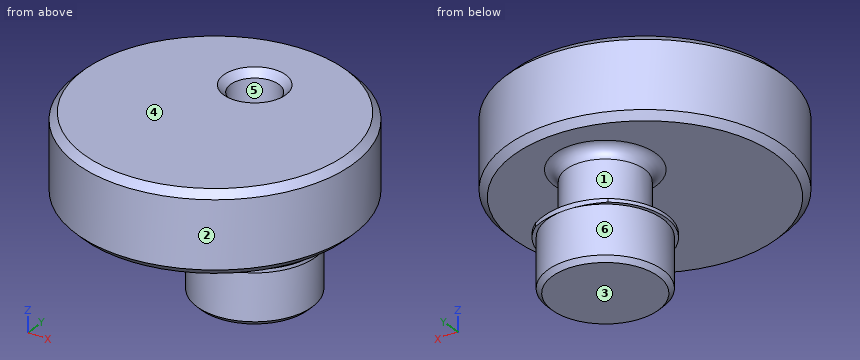
Autodesk Inventor part; units mm, degrees
ref_plane "YZ Plane" through (0, 0, 0) normal (1, 0, 0) x (0, 1, 0)
ref_plane "XZ Plane" through (0, 0, 0) normal (0, 1, 0) x (-1, 0, 0)
ref_plane "XY Plane" through (0, 0, 0) normal (0, 0, 1) x (1, 0, 0)
sketch "Sketch1" plane through (0, 0, 0) normal (0, 0, 1) x (1, 0, 0)
  circle A0 centre (0, 0) radius 6
  dimension "d0" = 12
extrude "Extrusion1" add sketch "Sketch1" along normal blind 3.5
sketch "Sketch2" plane through (0, 0, 3.5) normal (0, 0, 1) x (1, 0, 0)
  circle A0 centre (0, 2.5) radius 1.05
  line L0 (0, 2.5) -> (0, 0) construction
  dimension "d3" = 2.1
  dimension "d4" = 2.5
extrude "Extrusion2" add sketch "Sketch2" along normal blind 15 and the other way blind 8.25
chamfer "Chamfer1" distance 0.3 angle 45 2 edges at (-6, 0, 3.5) (-6, 0, 0)
sketch "Sketch4" plane through (0, 2.5, -4.75) normal (0, 0, -1) x (-1, 0, 0)
  circle A0 centre (0, 0) radius 1.05
  point P0 (0, -2.5)
extrude "Extrusion4" cut sketch "Sketch4" against normal through all
sketch "Sketch5" plane through (0, 0, 0) normal (1, 0, 0) x (0, 1, 0)
  line L0 (3.55, 0) -> (1.45, 0) construction
  line L1 (2.5, 0) -> (2.5, -4.1) construction
  line L2 (2.5, -5.1) -> (4.8, -5.1)
  line L3 (4.8, -5.1) -> (5, -4.9)
  line L4 (5, -4.9) -> (5, -2.8)
  line L5 (5, -2.8) -> (5.15, -2.8)
  line L6 (5.15, -2.8) -> (5.15, -2.65)
  line L7 (5.15, -2.65) -> (4.2, -2.3)
  line L8 (4.2, -2.3) -> (4.2, 0)
  line L9 (4.2, 0) -> (3.55, 0)
  line L10 (3.55, 0) -> (3.55, -4.1)
  line L11 (3.55, -4.1) -> (2.5, -4.1)
  line L12 (2.5, -4.1) -> (2.5, -5.1)
  line L13 (3.55, 0) -> (2.5, 0) construction
  point P0 (0, 0)
  dimension "d17" = 2.3
  dimension "d18" = 135
  dimension "d19" = 0.2
  dimension "d20" = 2.5
  dimension "d21" = 0.15
  dimension "d22" = 0.15
  dimension "d23" = 2.3
  dimension "d24" = 1.7
  dimension "d25" = 2.8
  dimension "d26" = 1
revolve "Revolution1" add sketch "Sketch5" angle 360 about axis through (0, 2.5, 0) along (0, 0, -1)
fillet "Fillet1" radius 0.5 1 edges at (0, 0.8, 0)
chamfer "Chamfer2" distance 0.3 angle 45 1 edges at (1.05, 2.5, 3.5)
sketch "Sketch6" plane through (0, 2.5, -2.8) normal (0, 0, -1) x (-1, 0, 0)
  circle A0 centre (0, -1) radius 3.5
  circle A1 centre (0, 0) radius 2.5
  circle A2 centre (0, 0) radius 2.65
  line L0 (0, 0) -> (0, -1) construction
  point P0 (0, -2.5)
  point P1 (1.5983, 2.1137)
  point P2 (-1.5983, 2.1137)
  dimension "d32" = 1
extrude "Extrusion5" cut sketch "Sketch6" against normal blind 1 contours A0 A2 picked at (0.1892, 2.5795)
properties part number "TestCam"
Part model, mm, in its own coordinate system. Face numbers are marked on the shaded views. A direction names the side the tool comes from. Give positions to 0.01 mm unless a question says otherwise; leave off trailing zeros. Loops run counter-clockwise (first coordinate to the right, second up) from the corner with the lowest first, then second, coordinate; pieces in that order, holes last.
(1) Drill centre lines: line 1 along X through (y, z) = (2.5, -1.75); line 2 along Y through (x, z) = (0, 1.25); line 3 along Z through (x, y) = (-0.75, -1.25). Where is each one in solid material? Low to high.
Return value:
line 1: x = -1.7 to -1.05, 1.05 to 1.7
line 2: y = -6 to 1.45, 3.55 to 6
line 3: z = 0 to 3.5
(2) Band-saw the part on A-A (z = -1). Write the cut outline in (x, y), and give its area (3 significant figures).
Return value:
outline: circle Ø3.4 at (0, 2.5); hole circle Ø2.1 at (0, 2.5)
area: 5.62 mm2
(3) Pull direction Z, two halves, no side cores. Call the marked faces 1, 2 and 3: pulls with the +Z half, pulls with the -Z half, needs draft (parallel to the pull), parting line crosses it, or undercut.
Return value:
face 1: undercut
face 2: needs draft
face 3: pulls with the -Z half
(4) 3-axis set-ups, long thin cutter, end or side, ignore diameter. For the marked faces 4, 5 and 6: which of +Z, -Z, +X, -X, +Y, -Y reach the whole face in a straight line?
Return value:
face 4: +Z, +X, -X, +Y, -Y
face 5: +Z
face 6: -Z
(5) Band-saw the part on B-B (z = -3). Write the cut outline in (x, y), and give its area (3 significant figures).
Return value:
outline: circle Ø5 at (0, 2.5); hole circle Ø2.1 at (0, 2.5)
area: 16.2 mm2
(6) Pin check, flat tips, straight feed: pin 1 (3 mm diameter, centred on x = 1.5, y = -3, fed in from -Z); pin 2 (1 mm diameter, centred on x = 0, y = 2.5, fed in from +Z); pin 3 (1.5 mm diameter, centred on x = 1.5, z = -1.5, fed in from -Y). Stop position of each tip, or through.
Return value:
pin 1: stops at z = 0
pin 2: stops at z = -4.1
pin 3: stops at y = 0.97
